Read the model definition and answer for the solid it produces. Units are mm, in the model's axes. Face numbers are marked on the shaded views. Coordinates: 2 decimals unless noted, no trailing zeros. Write each loop counter-clockwise with the first axis right and the second up, starting at its lowest first coordinate (ties: lowest second). Pieces come first, ordered by that corner, then holes. Notation, with made-up numbers: (9.25, 17.25) -> (51.25, 17.25) arc R26 ccw to (51.25, 38.25) -> close; hole circle Ø11 at (57, -1). An arc over 180 degrees is marked (long way). Answer as a JSON object with one key per item and string values. Group by question number.
(1) Find section D-D (z = 12.5). Give the vertices of the cut face in (x, y), then the cut area to 3 significant figures.
(2) Find section A-A (z = 4). Give the vertices of the cut face in (x, y).
(3) Straight lines are drawn through the part: L1, parallel to Z at x = -5.25, y = -0.05; L2, parallel to Z at x = 4, y = -0.55; L3, parallel to Z at x = 0, y = -0.6. For each, find the intervals that lie inside material, in ascending order.
(4) Find section B-B (x = -11.25). Give the vertices of the cut face in (y, z).
(5) Find section C-C (x = 0.25). Give the vertices of the cut face in (y, z), then the cut area to 3 significant figures.
(6) For a pull along Y with two mould halves and no side action, classify the marked faces 1 and 2 as +Y half, -Y half, draft (parallel to the pull), parting line (faces both ways), or undercut.
from build123d import *

# Parameters (mm, degrees)
F0_R     = 1
F1_DEPTH = 1.2
F2_R     = 2.15


# Not quite as in the source:
# - a feature names something its author has since deleted; it is built from what else it names


with BuildPart() as f1:
    # F0 (on Front) → F1 (new body)
    with BuildSketch(Plane.XZ):
        with BuildLine():
            ThreePointArc((-2.2, -11.3894688199), (0, 11.6), (2.2, -11.3894688199))
            Line((2.2, -11.3894688199), (2.2, -12.4894688199))
            ThreePointArc((2.2, -12.4894688199), (5.1370226671, -11.6633518005), (7.8168023095, -10.2048071338))
            ThreePointArc((7.8168023095, -10.2048071338), (0, 14.6), (-7.8168023095, -10.2048071338))
            ThreePointArc((-7.8168023095, -10.2048071338), (-5.1370226671, -11.6633518005), (-2.2, -12.4894688199))
            Line((-2.2, -12.4894688199), (-2.2, -11.3894688199))
        make_face()
        with BuildLine():
            ThreePointArc((7.8168023095, -10.2048071338), (5.1370226671, -11.6633518005), (2.2, -12.4894688199))
            Line((2.2, -12.4894688199), (2.2, -15.7894688199))
            ThreePointArc((2.2, -15.7894688199), (4.2270149149, -15.3713913009), (6.1827847392, -14.6942335113))
            Line((6.1827847392, -14.6942335113), (7.8168023095, -10.2048071338))
        make_face()
        with Locations((4.5011299048, -12.9922397434)):
            Circle(F0_R, mode=Mode.SUBTRACT)
        with BuildLine():
            Line((-2.2, -15.7894688199), (-2.2, -12.4894688199))
            ThreePointArc((-2.2, -12.4894688199), (-5.1370226671, -11.6633518005), (-7.8168023095, -10.2048071338))
            Line((-7.8168023095, -10.2048071338), (-6.1827847392, -14.6942335113))
            ThreePointArc((-6.1827847392, -14.6942335113), (-4.2270149149, -15.3713913009), (-2.2, -15.7894688199))
        make_face()
        with Locations((-4.5011299048, -12.9922397434)):
            Circle(F0_R, mode=Mode.SUBTRACT)
    extrude(amount=F1_DEPTH)

    # F2
    f2_edges = [f1.edges().sort_by_distance(p)[0] for p in [
        (6.182785, -0.6, -14.694234),
        (-6.182785, -0.6, -14.694234),
        (-7.816802, -0.6, -10.204807),
        (7.816802, -0.6, -10.204807),
    ]]
    fillet(f2_edges, radius=F2_R)


solid = f1.part
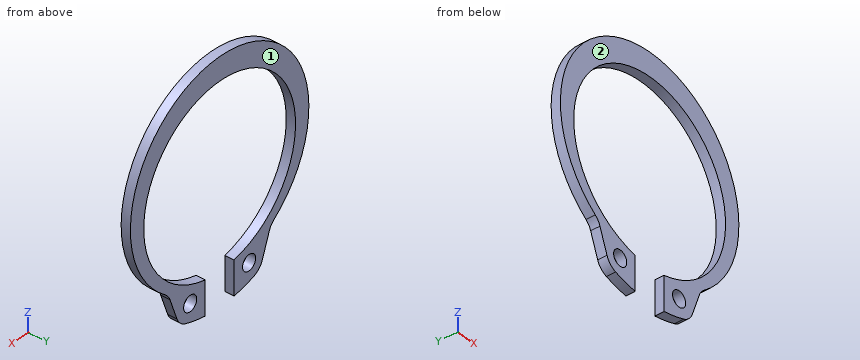
Results below:
{
 "1": {"outline": "(-7.27, -1.2) -> (7.27, -1.2) -> (7.27, 0) -> (-7.27, 0) -> close", "area": "17.4 mm2"},
 "2": {"outline": "(-13.29, -1.2) -> (-10.89, -1.2) -> (-10.89, 0) -> (-13.29, 0) -> close; (10.89, -1.2) -> (13.29, -1.2) -> (13.29, 0) -> (10.89, 0) -> close"},
 "3": {"L1": "z = -15.05 to -13.65, -12.33 to -10.34, 10.34 to 13.55", "L2": "z = -15.43 to -13.86, -12.13 to -10.89, 10.89 to 14", "L3": "z = 11.6 to 14.6"},
 "4": {"outline": "(-1.2, -6.74) -> (0, -6.74) -> (0, -2.83) -> (-1.2, -2.83) -> close; (-1.2, 2.83) -> (0, 2.83) -> (0, 8.67) -> (-1.2, 8.67) -> close"},
 "5": {"outline": "(-1.2, 11.6) -> (0, 11.6) -> (0, 14.6) -> (-1.2, 14.6) -> close", "area": "3.60 mm2"},
 "6": {"face 1": "+Y half", "face 2": "-Y half"}
}
